Model file for the job. Use its own axes, mm. A direction names the side the tool comes from. Round coordinates to 2 decimals unless told otherwise and drop trailing zeros. Loops run counter-clockwise (first coordinate to the right, second up) from the corner with the lowest first, then second, coordinate; pieces in that order, holes last. Notation, with made-up numbers: M 87.5,53 L 116.5,53 A20 ccw 116.5,58 Z; hole C 67,-11.5 d6. An arc over 180 degrees is marked long. Use a Markdown table: item, result. Add a question column.
Item 1: Saw through at D-D on x = 4. Write the cut outline in (y, z), then the cut area to 3 significant figures.
Item 2: Saw through at A-A on x = 20.5. Write the cut outline in (y, z).
Item 3: Saw through at C-C on y = 6. Write the cut outline in (x, z).
Item 4: Wall check: L1, parallel to Y at x = 17.75, z = 4.5; L2, parallel to Y at x = 4, z = 1.5; L3, parallel to X at y = 9, z = 1. Give the ranges that are in metal, low to high. Write a range as from..to.
Item 5: Two-plate mould, pull along Y, no slides. Class faces 1 (the flat face through (14, 22, 0)), 2 (the flat face through (10, 43, 3)), 3 (the cylindrical face through (0.41, 32.04, 3.45)): +Y half, -Y half, draft (parallel to the pull), parting line (faces both ways), or undercut.
Item 6: Saw through at B-B on z = 1. Write the cut outline in (x, y), then the cut area to 3 significant figures.
Item 7: Tool access for faces 4 (the cylindrical face through (24.793, 39.091, 3.451)), 5 (the cylindrical face through (0.434, 11.018, 3.451)): list every direction of +Z, -Z, +X, -X, +Y, -Y with a clear straight run to the whole face (end or side of a thin tool).
Item 8: Pin check, flat tips, straight feed: P1, Ø2, axis at y = 20.5, z = 5.5, coming from the -X side; P2, Ø1.8, axis at x = 4, y = 6, coming from the +Z side; P3, Ø1, axis at y = 11.5, z = 2, coming from the +X side; P4, Ø1, axis at y = 17.5, z = 4.5, coming from the -X side. Stop position of each tip, or through.
```python
from build123d import *

# Parameters (mm, degrees)
CROQUIS1_R              = 4
CROQUIS1_R_2            = 1.5
SALIENTE_EXTRUIR1_DEPTH = 7


with BuildPart() as part:
    # Croquis1 → Saliente-Extruir1 (new body)
    with BuildSketch(Plane.XY):
        with BuildLine():
            Line((5, 0), (15.5, 0))
            ThreePointArc((15.5, 0), (24.692388155, 3.807611845), (28.5, 13))
            Line((28.5, 13), (28.5, 30))
            ThreePointArc((28.5, 30), (24.692388155, 39.192388155), (15.5, 43))
            Line((15.5, 43), (5, 43))
            ThreePointArc((5, 43), (1.464466094, 41.535533906), (0, 38))
            Line((0, 38), (0, 34.019984026))
            ThreePointArc((0, 34.019984026), (0.422240466, 32.008984859), (1.617647059, 30.337635783))
            ThreePointArc((1.617647059, 30.337635783), (5.5, 21.5), (1.617647059, 12.662364217))
            ThreePointArc((1.617647059, 12.662364217), (0.422240466, 10.991015141), (0, 8.980015974))
            Line((0, 8.980015974), (0, 5))
            ThreePointArc((0, 5), (1.464466094, 1.464466094), (5, 0))
        make_face()
        with Locations((20.5, 31.5)):
            Circle(CROQUIS1_R, mode=Mode.SUBTRACT)
        with Locations((20.5, 11.5)):
            Circle(CROQUIS1_R, mode=Mode.SUBTRACT)
        with Locations((4, 37)):
            Circle(CROQUIS1_R_2, mode=Mode.SUBTRACT)
        with Locations((4, 6)):
            Circle(CROQUIS1_R_2, mode=Mode.SUBTRACT)
    extrude(amount=SALIENTE_EXTRUIR1_DEPTH)


solid = part.part
```
Entries:
| question | item | result |
|---|---|---|
| 1 | outline | M 0.1,0 L 4.5,0 L 4.5,7 L 0.1,7 Z; M 7.5,0 L 15.69,0 L 15.69,7 L 7.5,7 Z; M 27.31,0 L 35.5,0 L 35.5,7 L 27.31,7 Z; M 38.5,0 L 42.9,0 L 42.9,7 L 38.5,7 Z |
| 1 | area | 176 mm2 |
| 2 | outline | M 1,0 L 7.5,0 L 7.5,7 L 1,7 Z; M 15.5,0 L 27.5,0 L 27.5,7 L 15.5,7 Z; M 35.5,0 L 42,0 L 42,7 L 35.5,7 Z |
| 3 | outline | M 0,0 L 2.5,0 L 2.5,7 L 0,7 Z; M 5.5,0 L 26.45,0 L 26.45,7 L 5.5,7 Z |
| 4 | L1 | 0.2..8.6, 14.4..28.6, 34.4..42.8 |
| 4 | L2 | 0.1..4.5, 7.5..15.69, 27.31..35.5, 38.5..42.9 |
| 4 | L3 | 0..17.38, 23.62..27.87 |
| 5 | face 1 | draft |
| 5 | face 2 | +Y half |
| 5 | face 3 | undercut |
| 6 | outline | M 0,5 A5 ccw 5,0 L 15.5,0 A13 ccw 28.5,13 L 28.5,30 A13 ccw 15.5,43 L 5,43 A5 ccw 0,38 L 0,34.02 A5 ccw 1.62,30.34 A12 cw 1.62,12.66 A5 ccw 0,8.98 Z; hole C 4,6 d3; hole C 4,37 d3; hole C 20.5,11.5 d8; hole C 20.5,31.5 d8 |
| 6 | area | 948 mm2 |
| 7 | face 4 | +Z, -Z, +X, +Y |
| 7 | face 5 | +Z, -Z, -X |
| 8 | P1 | x = 5.33 |
| 8 | P2 | through |
| 8 | P3 | x = 28.46 |
| 8 | P4 | x = 4.62 |
